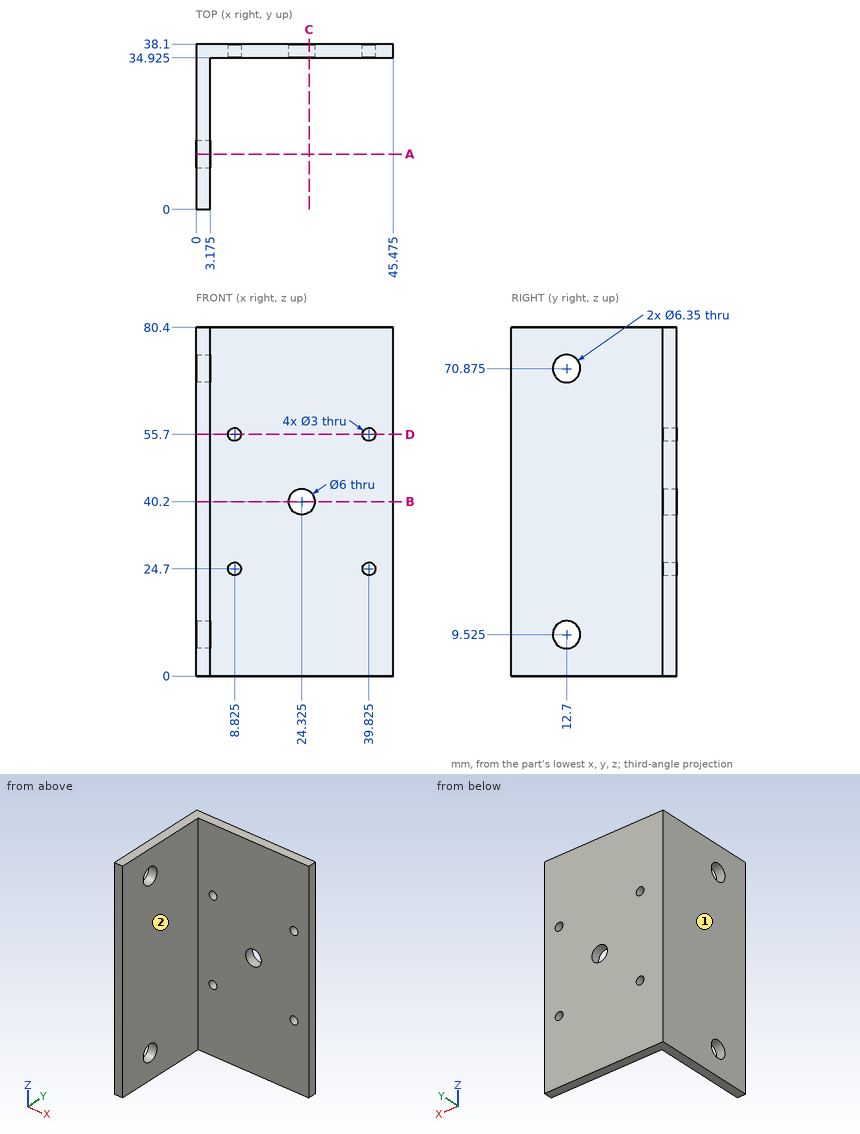
The drawing under review shows one solid part. Ordinate dimensions are in mm from its lowest x, y, z. A direction names the side the tool comes from. Round coordinates to 2 decimals unless told otherwise and drop trailing zeros. Order: outer loops, then holes, each group sorted by start corner. A loop starts at its lowest first (then second) coordinate and runs counter-clockwise, first axis right, second up. Notation, with made-up numbers: (76.5, 0) -> (104.5, 0) arc R21 cw to (104.5, 25) -> close; hole circle Ø5 at (8, -29.5). An arc over 180 degrees is marked (long way). Return JSON: item names as keys, results as strings.
1. For L1, parallel to X at y = 37, z = 24.7 (3 decimals); L2, parallel to X at y = 36, z = 40 (3 decimals); L3, parallel to Y at x = 12.5, z = 34.5 (3 decimals), list the stretches that pass through material, from the lowest coordinate up. Write a range as [from, to].
Answer block:
{"L1": "x = [0, 7.325], [10.325, 38.325], [41.325, 45.475]", "L2": "x = [0, 21.332], [27.318, 45.475]", "L3": "y = [34.925, 38.1]"}
2. Insertion check: P1, Ø5.5, axis at y = 12.7, z = 70.875, coming from the -X side; P2, Ø8, axis at y = 20.5, z = 16.5, coming from the -X side; P3, Ø1.5, axis at x = 35.5, z = 57.5, coming from the -Y side (3 decimals); P4, Ø6, axis at y = 8, z = 15, coming from the +X side (3 decimals). Each pin has a flat end and moves straight along its axis. Give the tip position at first contact, or say it passes through.
Answer block:
{"P1": "passes through", "P2": "stops at x = 0", "P3": "stops at y = 34.925", "P4": "stops at x = 3.175"}
3. Take a section at C-C (x = 26). Write out the cut boundary in (y, z) (3 decimals).
Answer block:
{"outline": "(34.925, 0) -> (38.1, 0) -> (38.1, 37.711) -> (34.925, 37.711) -> close; (34.925, 42.689) -> (38.1, 42.689) -> (38.1, 80.4) -> (34.925, 80.4) -> close"}
4. Take a section at A-A (y = 12.7). Write out the cut boundary in (x, z) (3 decimals), then the cut area to 3 significant figures.
Answer block:
{"outline": "(0, 0) -> (3.175, 0) -> (3.175, 6.35) -> (0, 6.35) -> close; (0, 12.7) -> (3.175, 12.7) -> (3.175, 67.7) -> (0, 67.7) -> close; (0, 74.05) -> (3.175, 74.05) -> (3.175, 80.4) -> (0, 80.4) -> close", "area": "215 mm²"}
5. Take a section at D-D (z = 55.7). Write out the cut boundary in (x, y) (3 decimals), then the cut area to 3 significant figures.
Answer block:
{"outline": "(0, 0) -> (3.175, 0) -> (3.175, 34.925) -> (7.325, 34.925) -> (7.325, 38.1) -> (0, 38.1) -> close; (10.325, 34.925) -> (38.325, 34.925) -> (38.325, 38.1) -> (10.325, 38.1) -> close; (41.325, 34.925) -> (45.475, 34.925) -> (45.475, 38.1) -> (41.325, 38.1) -> close", "area": "236 mm²"}
6. Take a section at B-B (z = 40.2). Write out the cut boundary in (x, y) (3 decimals).
Answer block:
{"outline": "(0, 0) -> (3.175, 0) -> (3.175, 34.925) -> (21.325, 34.925) -> (21.325, 38.1) -> (0, 38.1) -> close; (27.325, 34.925) -> (45.475, 34.925) -> (45.475, 38.1) -> (27.325, 38.1) -> close"}
7. For the marked faces 1 and 2, list the 3-axis set-ups (+Z, -Z, +X, -X, +Y, -Y) from which the entire face can be reached by the end or side of a thin tool; tool diameter is ignored.
Answer block:
{"face 1": "+Z, -Z, -X, +Y, -Y", "face 2": "+Z, -Z, +X, -Y"}
